Could you check a few things on this drawing? It's one solid part, dimensions in mm from its lowest x, y, z. A direction names the side the tool comes from. Round coordinates to 2 decimals unless told otherwise and drop trailing zeros. Loops run counter-clockwise (first coordinate to the right, second up) from the corner with the lowest first, then second, coordinate; pieces in that order, holes last. Notation, with made-up numbers: M 20,78 L 77,78 A34 ccw 77,113 Z; hole C 35,77.25 d8. An arc over 180 degrees is marked long. Put each result on its own line as item: value. Start each with the question number.
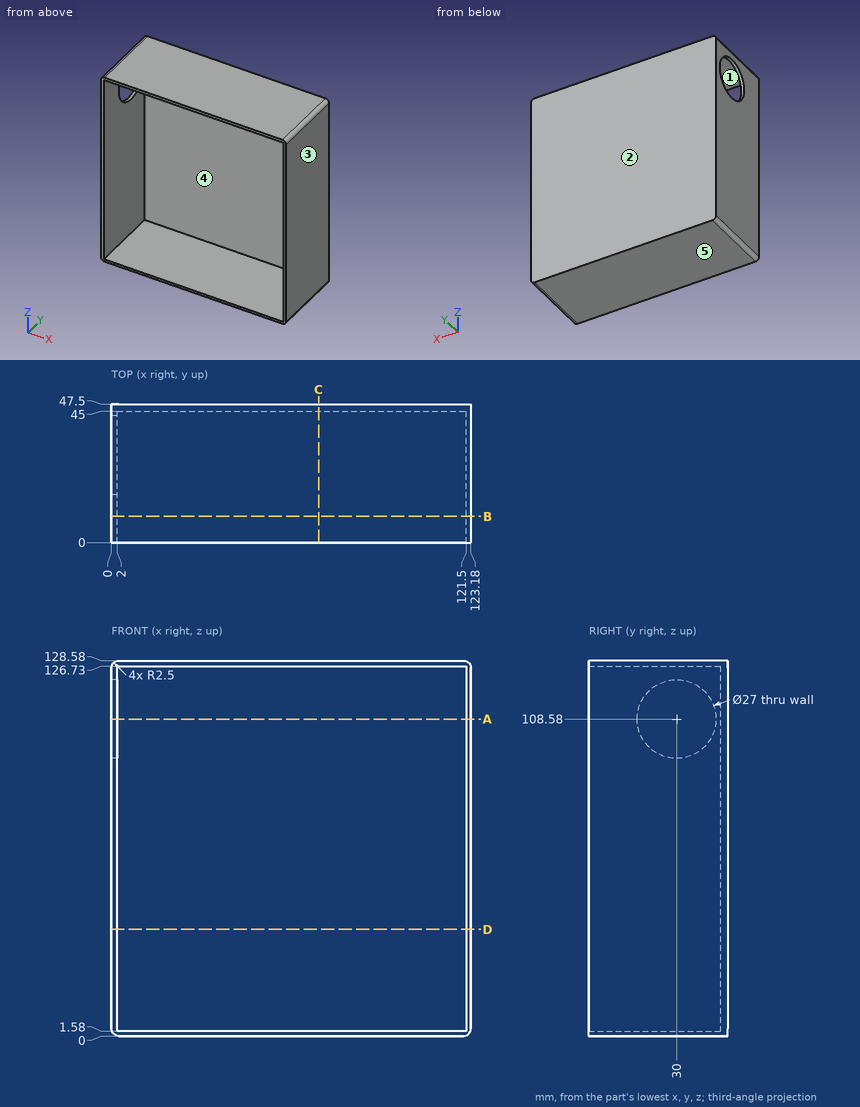
1) Suppose I cut it at C-C (x = 71). Write out the boundary of the cut face in (y, z), plus the area to 3 significant figures.
2) Suppose I cut it at A-A (z = 108.58). Write out the boundary of the cut face in (x, y), plus the area to 3 significant figures.
3) If I drill on probe 1 along X at (y, z) = (37, 89.5); probe 2 along Z at (x, y) = (41, 27); probe 3 along Y at (x, z) = (94, 81.5), over which ranges is the centre line in solid material (lowest first)? Write a range as from..to.
4) I'm going to push flat-ended pins straight in: P1, Ø22.5, axis at x = 38.5, y = 30.5, coming from the -Z side; P2, Ø10, axis at x = 56.5, z = 48, coming from the -Y side. Where does each tip first touch, or does it pass through?
5) Suppose I cut it at D-D (z = 36.5). Write out the boundary of the cut face in (x, y), plus the area to 3 significant figures.
6) Suppose I cut it at B-B (y = 9). Write out the boundary of the cut face in (x, z), plus the area to 3 significant figures.
7) On a 3-axis mill with a long thin cutter (end or side, diameter ignored), from which of +Z, -Z, +X, -X, +Y, -Y can I reach the whole of each face in a straight line? I mean the marked faces 1 and 2. Say none if no direction works.
8) If we mould it in two halves opening along Z, with no side actions, what happens to the marked faces 3, 4 and 5? For each: pulls with the +Z half, pulls with the -Z half, needs draft (parallel to the pull), parting line crosses it, or undercut.
Results are:
1. outline: M 0,0 L 47.5,0 L 47.5,128.58 L 0,128.58 L 0,126.73 L 45,126.73 L 45,1.58 L 0,1.58 Z
1. area: 476 mm²
2. outline: M 0,0 L 2,0 L 2,16.5 L 0,16.5 Z; M 0,43.5 L 2,43.5 L 2,45 L 121.5,45 L 121.5,0 L 123.18,0 L 123.18,47.5 L 0,47.5 Z
2. area: 420 mm²
3. probe 1: 0..2, 121.5..123.18
3. probe 2: 0..1.58, 126.73..128.58
3. probe 3: 45..47.5
4. P1: z = 0
4. P2: y = 45
5. outline: M 0,0 L 2,0 L 2,45 L 121.5,45 L 121.5,0 L 123.18,0 L 123.18,47.5 L 0,47.5 Z
5. area: 474 mm²
6. outline: M 0,2.5 A2.5 ccw 2.5,0 L 120.68,0 A2.5 ccw 123.18,2.5 L 123.18,126.08 A2.5 ccw 120.68,128.58 L 2.5,128.58 A2.5 ccw 0,126.08 Z; hole M 2,1.58 L 121.5,1.58 L 121.5,126.73 L 2,126.73 Z
6. area: 878 mm²
7. face 1: -Y
7. face 2: +Z, -Z, +X, -X, +Y
8. face 3: needs draft
8. face 4: undercut
8. face 5: pulls with the -Z half
